Here's how the part is built. I have some questions about the finished solid (model axes, mm). Face numbers are marked on the shaded views. A direction names the side the tool comes from. Round coordinates to 2 decimals unless told otherwise and drop trailing zeros. Loops run counter-clockwise (first coordinate to the right, second up) from the corner with the lowest first, then second, coordinate; pieces in that order, holes last. Notation, with made-up numbers: (87.5, 88.25) - (92.5, 88.25) arc R25 ccw to (92.5, 118.25) - close; hole circle Ø3 at (-38, -9). An arc over 180 degrees is marked (long way). Answer as a JSON object with one key per item and string values. Group by question number.
1) I want a section at C-C, the plane y = 4.25. Please give me the cut outline in (x, z), then the cut area to 3 significant figures.
2) I want a section at D-D, the plane z = 29. Please give me the cut outline in (x, y).
3) Will these pins go through, and if not, where does the flat tip stop? P1, Ø1.5, axis at x = -13.5, y = 3.5, coming from the +Z side; P2, Ø5, axis at y = 3.5, z = 29.5, coming from the -X side; P3, Ø3, axis at x = -23, y = 4, coming from the -Z side.
4) If I drill on line 1 along Z through (x, y) = (-15, 5.5); line 2 along X through (y, z) = (2.5, 0.5); line 3 along Y through (x, z) = (-1, -29), over which ranges is the centre line in solid material (lowest first)? Write a range as [from, to].
5) Which directions (+Z, -Z, +X, -X, +Y, -Y) give clear straight access to the entire face, cutting with the end or side of a thin tool? Please do the marked faces 1 and 2.
6) If we mould it in two halves opening along X, with no side actions, what happens to the marked faces 3, 4 and 5? For each: pulls with the +X half, pulls with the -X half, needs draft (parallel to the pull), parting line crosses it, or undercut.
7) I want a section at B-B, the plane x = -15. Please give me the cut outline in (y, z), then the cut area to 3 significant figures.
8) I want a section at A-A, the plane z = 0. Please give me the cut outline in (x, y).
Autodesk Inventor part; units mm, degrees
ref_plane "YZ Plane" through (0, 0, 0) normal (1, 0, 0) x (0, 1, 0)
ref_plane "XZ Plane" through (0, 0, 0) normal (0, 1, 0) x (-1, 0, 0)
ref_plane "XY Plane" through (0, 0, 0) normal (0, 0, 1) x (1, 0, 0)
sketch "Sketch1" plane through (0, 0, 0) normal (0, 1, 0) x (-1, 0, 0)
  line L0 (4, 35) -> (-4, 35)
  line L1 (-4, 35) -> (-4, -35)
  line L2 (-4, -35) -> (4, -35)
  line L3 (4, -35) -> (4, 35)
  line L4 (4, 35) -> (-4, -35) construction
  line L5 (-4, 35) -> (4, -35) construction
  circle A0 centre (15, 0) radius 15
  arc A1 (4, 22.2261) -> (12.6667, 14.8174) centre (11.5, 22.2261) ccw
  arc A2 (12.6667, -14.8174) -> (4, -22.2261) centre (11.5, -22.2261) ccw
  point P0 (0, 0)
  dimension "d0" = 8
  dimension "d1" = 70
  dimension "d2" = 30
  dimension "d3" = 15
  dimension "d6" = 15
  dimension "d7" = 7.5
  dimension "d9" = 0
  dimension "d10" = 15
extrude "Extrusion1" add sketch "Sketch1" along normal blind 10
sketch "Sketch2" plane through (0, 10, 0) normal (0, 1, 0) x (1, 0, 0)
  circle A0 centre (-15, 0) radius 11.25
  arc A1 (-12.6667, 14.8174) -> (-12.6667, -14.8174) centre (-15, 0) ccw
  point P0 (0, 0)
  dimension "d13" = 22.5
extrude "Extrusion2" cut sketch "Sketch2" against normal blind 7
sketch "Sketch3" plane through (-15, 3, 0) normal (0, 1, 0) x (1, 0, 0)
  circle A0 centre (0, 0) radius 10.5
  point P0 (15, 0)
  dimension "d16" = 21
extrude "Extrusion3" cut sketch "Sketch3" against normal blind 7
sketch "Sketch4" plane through (-4, 0, 22.2261) normal (-1, 0, 0) x (0, 0, 1)
  circle A0 centre (6.7739, 5) radius 3
  line L0 (0, 0) -> (12.7739, 0)
  line L1 (12.7739, 0) -> (12.7739, 10)
  circle A1 centre (-51.2261, 5) radius 3
  line L2 (-57.2261, 10) -> (-44.4522, 10)
  line L3 (-57.2261, 0) -> (-57.2261, 10)
  point P0 (-22.2261, 0)
  point P1 (6.3869, 0)
  dimension "d19" = 6
  dimension "d20" = 5
  dimension "d21" = 6
  dimension "d22" = 6
  dimension "d23" = 5
  dimension "d24" = 6
extrude "Extrusion4" cut sketch "Sketch4" against normal blind 7
properties part number "Bearing Holder"
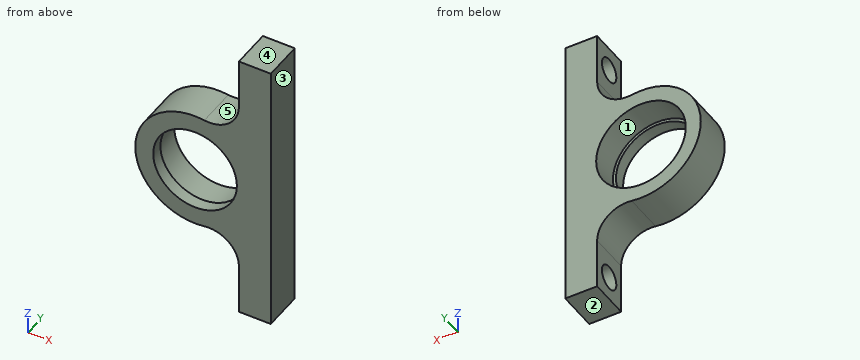
Outcome:
{
 "1": {"outline": "(-12.67, -14.82) arc R7.5 cw to (-4, -22.23) - (-4, -26.1) - (3, -26.1) - (3, -31.9) - (-4, -31.9) - (-4, -35) - (4, -35) - (4, 35) - (-4, 35) - (-4, 31.9) - (3, 31.9) - (3, 26.1) - (-4, 26.1) - (-4, 22.23) arc R7.5 cw to (-12.67, 14.82) arc R15 ccw (long way) to start; hole circle Ø22.5 at (-15, 0)", "area": "784 mm^2"},
 "2": {"outline": "(-4, 0) - (4, 0) - (4, 10) - (-4, 10) - (-4, 8) - (3, 8) - (3, 2) - (-4, 2) - close"},
 "3": {"P1": "z = 14.98", "P2": "x = -4", "P3": "z = -13.52"},
 "4": {"line 1": "[-15, -11.25], [11.25, 15]", "line 2": "[-29.99, -25.49], [-4.51, 4]", "line 3": "[0, 2], [8, 10]"},
 "5": {"face 1": "+Y", "face 2": "-Z, +X, -X, +Y, -Y"},
 "6": {"face 3": "pulls with the +X half", "face 4": "needs draft", "face 5": "undercut"},
 "7": {"outline": "(0, -15) - (10, -15) - (10, -11.25) - (3, -11.25) - (3, -10.5) - (0, -10.5) - close; (0, 10.5) - (3, 10.5) - (3, 11.25) - (10, 11.25) - (10, 15) - (0, 15) - close", "area": "79.5 mm^2"},
 "8": {"outline": "(-30, 0) - (-25.5, 0) - (-25.5, 3) - (-26.25, 3) - (-26.25, 10) - (-30, 10) - close; (-4.5, 0) - (4, 0) - (4, 10) - (-3.75, 10) - (-3.75, 3) - (-4.5, 3) - close"}
}
